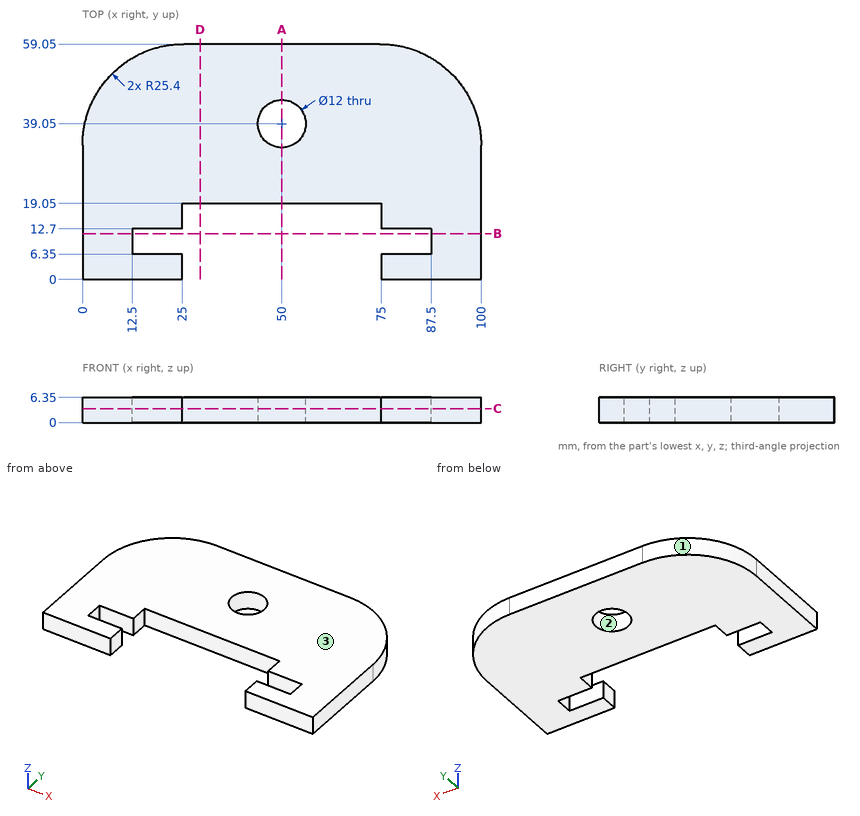
Geometry: see drawing. Coordinates: mm, zero at the bounding-box minimum. Give positions to 0.01 mm unless a question says otherwise; leave off trailing zeros. Loops run counter-clockwise (first coordinate to the right, second up) from the corner with the lowest first, then second, coordinate; pieces in that order, holes last. Notation, with made-up numbers: (59, 25.5) - (92, 25.5) arc R22 cw to (92, 52.5) - close; hole circle Ø10 at (-13, -12). An arc over 180 degrees is marked (long way). One line per question, with ' | ' between items. Start each with the question number.
(1) Section query B-B on y = 11.5. Return loops of the section in (x, z).
(2) Section query D-D on x = 29.5. Return loops of the section in (y, z), then the cut area to 3 significant figures.
(3) Section query C-C on z = 3.5. Return loops of the section in (x, y), then the cut area to 3 significant figures.
(4) Contact query for flat-ended pins moving along their axis: pin 1 (12 mm diameter, centred on x = 16, y = 47, fed in from -Z); pin 2 (1.9 mm diameter, centred on x = 42.5, z = 2.5, fed in from -Y). Output: stop coordinate, or through.
(5) Ray query, line 1 (Y direction, x = 50, z = 2); line 2 (X direction, y = 11, z = 6.25); line 3 (X direction, y = 18, z = 2). Return the intervals inside material, ascending. Write a range as from..to.
(6) Pull-direction query (X, two-part tool) for the marked faces 1, 2 and 3; classes: released by +X, released by -X, zero draft, split by the parting line, or undercut.
(7) Section query A-A on x = 50. Return loops of the section in (y, z).
The answers:
1) outline: (0, 0) - (12.5, 0) - (12.5, 6.35) - (0, 6.35) - close; (87.5, 0) - (100, 0) - (100, 6.35) - (87.5, 6.35) - close
2) outline: (19.05, 0) - (59.05, 0) - (59.05, 6.35) - (19.05, 6.35) - close | area: 254 mm2
3) outline: (0, 0) - (25, 0) - (25, 6.35) - (12.5, 6.35) - (12.5, 12.7) - (25, 12.7) - (25, 19.05) - (75, 19.05) - (75, 12.7) - (87.5, 12.7) - (87.5, 6.35) - (75, 6.35) - (75, 0) - (100, 0) - (100, 33.65) arc R25.4 ccw to (74.6, 59.05) - (25.4, 59.05) arc R25.4 ccw to (0, 33.65) - close; hole circle Ø12 at (50, 39.05) | area: 4,400 mm2
4) pin 1: z = 0 | pin 2: y = 19.05
5) line 1: 19.05..33.05, 45.05..59.05 | line 2: 0..12.5, 87.5..100 | line 3: 0..25, 75..100
6) face 1: released by -X | face 2: undercut | face 3: zero draft
7) outline: (19.05, 0) - (33.05, 0) - (33.05, 6.35) - (19.05, 6.35) - close; (45.05, 0) - (59.05, 0) - (59.05, 6.35) - (45.05, 6.35) - close
